Autodesk Inventor part; units mm, degrees
ref_plane "YZ Plane" through (0, 0, 0) normal (1, 0, 0) x (0, 1, 0)
ref_plane "XZ Plane" through (0, 0, 0) normal (0, 1, 0) x (-1, 0, 0)
ref_plane "XY Plane" through (0, 0, 0) normal (0, 0, 1) x (1, 0, 0)
sketch "Sketch1" plane through (0, 0, 0) normal (0, 1, 0) x (-1, 0, 0)
  circle A0 centre (-6.6375, -88.2502) radius 58
  line L0 (-14.6375, 98.7498) -> (-14.6375, -12.6724)
  arc A1 (-14.6375, -12.6724) -> (-73.5777, -52.264) centre (-6.6375, -88.2502) ccw
  line L1 (-73.5777, -52.264) -> (-112.0003, 98.7498)
  line L2 (-112.0003, 98.7498) -> (-14.6375, 98.7498)
  line L3 (98.7253, 98.7498) -> (60.3027, -52.264)
  arc A2 (60.3027, -52.264) -> (1.3625, -12.6724) centre (-6.6375, -88.2502) ccw
  line L4 (1.3625, -12.6724) -> (1.3625, 98.7498)
  line L5 (1.3625, 98.7498) -> (98.7253, 98.7498)
  line L6 (67.0159, -106.9899) -> (119.3625, 98.7498)
  line L7 (119.3625, 98.7498) -> (119.3625, 131.7498)
  line L8 (119.3625, 131.7498) -> (-132.6375, 131.7498)
  line L9 (-132.6375, 131.7498) -> (-132.6375, 98.7498)
  line L10 (-132.6375, 98.7498) -> (-80.2909, -106.9899)
  arc A3 (-80.2909, -106.9899) -> (67.0159, -106.9899) centre (-6.6375, -88.2502) ccw
extrude "Extrusion1" add sketch "Sketch1" along normal blind 15 contours A0 | L0 A1 L1 L2 | L3 A2 L4 L5 | A3 L10 L9 L8 L7 L6
chamfer "Chamfer1" distance 33 angle 45 2 edges at (-119.3625, 7.5, 131.7498) (132.6375, 7.5, 131.7498)
sketch "Sketch4" plane through (0, 15, 0) normal (0, 1, 0) x (1, 0, 0)
  line L0 (132.6375, -98.7498) -> (99.6375, -131.7498)
  line L1 (132.6375, -98.7498) -> (80.2909, 106.9899)
  arc A0 (80.2909, 106.9899) -> (-67.0159, 106.9899) centre (6.6375, 88.2502) ccw
  line L2 (-67.0159, 106.9899) -> (-119.3625, -98.7498)
  line L3 (-86.3625, -131.7498) -> (-119.3625, -98.7498)
  line L4 (-86.3625, -131.7498) -> (99.6375, -131.7498)
  line L5 (-97.308, -131.7498) -> (123, -131.7498)
  line L6 (123, -131.7498) -> (123, -121.7498)
  line L7 (123, -121.7498) -> (-97.308, -121.7498)
  line L8 (-97.308, -121.7498) -> (-97.308, -131.7498)
  line L9 (-122.7338, -105.2498) -> (137.8877, -105.2498)
  line L10 (137.8877, -105.2498) -> (137.8877, -95.2498)
  line L11 (137.8877, -95.2498) -> (-122.7338, -95.2498)
  line L12 (-122.7338, -95.2498) -> (-122.7338, -105.2498)
  point P0 (0, 0)
  point P1 (109.6375, -121.7498)
  point P2 (-96.3625, -121.7498)
  point P3 (131.747, -95.2498)
  point P4 (-118.472, -95.2498)
  point P5 (-118.8536, -96.7498)
  point P6 (132.1287, -96.7498)
  point P7 (-112.8625, -105.2498)
  point P8 (126.1375, -105.2498)
  dimension "d5" = 10
  dimension "d6" = 10
  dimension "d7" = 16.5
extrude "Extrusion2" add sketch "Sketch4" along normal blind 30 contours L0 L9 L3 L2 L11 L1 | L0 L4 L3 L7
sketch "Sketch5" plane through (-86.3625, 0, 131.7498) normal (0, 0, 1) x (1, 0, 0)
  line L0 (196, 45) -> (-10, 45)
  line L1 (0, 0) -> (186, 0)
  line L2 (60.5, 45) -> (125.5, 45)
  line L3 (125.5, 45) -> (125.5, 0)
  line L4 (125.5, 0) -> (60.5, 0)
  line L5 (60.5, 0) -> (60.5, 45)
  line L6 (186, 45) -> (186, 0)
  line L7 (0, 0) -> (0, 45)
  point P0 (86.3625, 0)
  point P1 (186, 22.5)
  point P2 (0, 22.5)
  dimension "d10" = 65
  dimension "d11" = 60.5
  dimension "d12" = 60.5
extrude "Extrusion3" cut sketch "Sketch5" against normal blind 4 contours L3 L1 L5 L0
properties part number "KrovatkaShatunFlanec" material "Aluminum 6061-AHC"
Could you check a few things on this model? Use its own coordinates, in mm. A direction names the side the tool comes from. Round coordinates to 2 decimals unless told otherwise and drop trailing zeros. Loops run counter-clockwise (first coordinate to the right, second up) from the corner with the lowest first, then second, coordinate; pieces in that order, holes last. Notation, with made-up numbers: M 3.5,1 L 8.5,1 A24 cw 8.5,18 Z; hole C 2.25,-14 d9. An arc over 180 degrees is marked long. Write item = value, one per line.
1. Will these pins go through, and if not, where does the flat tip stop? P1, Ø2, axis at y = 12.5, z = 130.5, coming from the -X side; P2, Ø10, axis at x = 54, y = 18.5, coming from the -Z side; P3, Ø9, axis at x = -9.5, y = 36, coming from the -Z side.
Results below:
P1 = -88.61
P2 = -150.37
P3 = 95.25
2. I need wall thicknesses on probe 1 along Z at (x, y) = (-64.5, 15.5); probe 2 along Z at (x, y) = (-92, 37.5); probe 3 along Y at (x, z) = (-4, -63). Which ranges of each line are inside material? Lowest first, please.
Results below:
probe_1 = 95.25 to 105.25, 121.75 to 131.75
probe_2 = 95.25 to 105.25, 121.75 to 126.11
probe_3 = 0 to 15
3. I want a section at D-D, the plane z = -73.5. Write out the boundary of the cut face in (x, y), and give its area (3 significant figures).
Results below:
outline = M -75.54,0 L 88.81,0 L 88.81,15 L -75.54,15 Z
area = 2,470 mm²
4. Which directions (+Z, -Z, +X, -X, +Y, -Y) give clear straight access to the entire face, cutting with the end or side of a thin tool? Please do faces 1 (the face through (-91.29, 29.79, 126.82)), 2 (the face through (8, 30, 95.25)), 3 (the face through (8, 15, 112)).
Results below:
face_1 = +Z, -X, +Y, -Y
face_2 = -Z, +X, -X, +Y
face_3 = +X, -X, +Y
5. I want a section at C-C, the plane x = -49.5. Write out the boundary of the cut face in (y, z).
Results below:
outline = M 0,-139.48 L 15,-139.48 L 15,95.25 L 45,95.25 L 45,105.25 L 15,105.25 L 15,121.75 L 45,121.75 L 45,131.75 L 0,131.75 Z
6. Thinking about a two-plate mould opening in Z: for faces 4 (the face through (5, 30, 105.25)), 5 (the face through (108.525, 10.728, 3.98)), 6 (the face through (115.91, 7.4, 115.48)), 7 (the face through (8, 15, -4)), which applies, +Z half, -Z half, draft (parallel to the pull), parting line (faces both ways), or undercut?
Results below:
face_4 = undercut
face_5 = -Z half
face_6 = +Z half
face_7 = draft
7. I want a section at A-A, the plane y = 34. Write out the boundary of the cut face in (x, z).
Results below:
outline = M -119.36,98.75 L -118.47,95.25 L 131.75,95.25 L 132.64,98.75 L 126.14,105.25 L -112.86,105.25 Z; M -96.36,121.75 L 109.64,121.75 L 99.64,131.75 L 39.14,131.75 L 39.14,127.75 L -25.86,127.75 L -25.86,131.75 L -86.36,131.75 Z
